Could you check a few things on this model? Use its own coordinates, in mm. A direction names the side the tool comes from. Give positions to 0.01 mm unless a question says otherwise; leave off trailing zeros. Loops run counter-clockwise (first coordinate to the right, second up) from the corner with the lowest first, then second, coordinate; pieces in that order, holes last. Notation, with made-up numbers: M 39,40.5 L 47,40.5 A18 cw 47,75.5 Z; hole C 47,30 d7. An arc over 180 degrees is marked long. Answer in a Markdown table with one row per item. Add a question column.
1. Thinking about a two-plate mould opening in Z: for faces 6 (the flat face through (33, 9, 10)), 7 (the flat face through (3.25, -3.31, 6.04)), 8 (the cylindrical face through (-17.257, -10.412, 5.594)), which applies, released by +Z, released by -Z, zero draft, split by the parting line, or undercut?
2. I'm going to push flat-ended pins straight in: pin 1 Ø3 at (y, z) = (-10, 8) entering from -X; pin 2 Ø5 at (y, z) = (1, 8.5) entering from -X; pin 3 Ø3 at (x, z) = (86, 4.5) entering from +Y. Where does each tip first touch, or does it pass through?
3. Which directions (+Z, -Z, +X, -X, +Y, -Y) give clear straight access to the entire face, cutting with the end or side of a thin tool? Please do faces 1 (the flat face through (-16, -12.947, 5)), 2 (the flat face through (6.1, 10.253, 6.3)), 3 (the flat face through (-19.9, -7.947, 3.8)), 4 (the flat face through (34, 6.053, 5)), 5 (the flat face through (86, -7.947, 3)).
4. If we section it at B-B on x = 17.5: List the corners of the cut face in (y, z) for me, then the cut area to 3 significant figures.
5. If we section it at C-C on y = 8.75: List the corners of the cut face in (x, z) for me, then the cut area to 3 significant figures.
6. I need wall thicknesses on line 1 along X through (y, z) = (-11.1, 5) (3 decimals); line 2 along X through (y, z) = (10.95, 5); line 3 along X through (y, z) = (7.5, 3.75). Which ranges of each line are inside material? Lowest first, please. Write a range as from..to.
7. If we section it at A-A on y = -9.5: List the corners of the cut face in (x, z) for me, then the cut area to 3 significant figures.
8. If we section it at D-D on z = 5: Count the separate pieces of the cut face and the enclosed holes in it, then the cut area to 3 significant figures.
```python
from build123d import *

# Parameters (mm, degrees)
EXTRUDE_1_DEPTH     = 10
SKETCH_2_R          = 1.6
CUT_EXTRUDE_2_DEPTH = 27
SKETCH_3_R          = 3.1
CUT_EXTRUDE_3_DEPTH = 2.8
SKETCH_5_R          = 1.55
CUT_EXTRUDE_4_DEPTH = 6


with BuildPart() as part:
    # 草图1 → 凸台-拉伸1 (new body)
    with BuildSketch(Plane.XY):
        Polygon((-3.188712924, 13.052848472), (33.811287076, 13.052848472), (33.811287076, 6.052848472), (16.311287076, 6.052848472), (-10.188712924, -12.947151528), (-26.188712924, -12.947151528), (-23.688712924, -7.947151528), (-13.688712924, -7.947151528), align=None)
    extrude_1 = extrude(amount=EXTRUDE_1_DEPTH)

    # 镜向1: 凸台-拉伸1 across plane
    add(extrude_1.mirror(Plane(origin=(33.811287076, 13.052848472, 10), x_dir=(0, 0, 1), z_dir=(-1, 0, 0))))

    # 草图2 → 切除-拉伸2 (cut, through all)
    with BuildSketch(Plane(origin=(0, 13.052848472, 0), x_dir=(1, 0, 0), z_dir=(0, 1, 0))):
        with Locations((4.811287076, -5)):
            Circle(SKETCH_2_R)
        with Locations((62.811287076, -5)):
            Circle(SKETCH_2_R)
    extrude(amount=-CUT_EXTRUDE_2_DEPTH, mode=Mode.SUBTRACT)

    # 草图3 → 切除-拉伸3 (cut)
    with BuildSketch(Plane(origin=(0, 13.052848472, 0), x_dir=(1, 0, 0), z_dir=(0, 1, 0))):
        with Locations((4.811287076, -5)):
            Circle(SKETCH_3_R)
        with Locations((62.811287076, -5)):
            Circle(SKETCH_3_R)
    extrude(amount=-CUT_EXTRUDE_3_DEPTH, mode=Mode.SUBTRACT)

    # 草图5 → 切除-拉伸4 (cut, through all)
    with BuildSketch(Plane(origin=(0, -7.947151528, 0), x_dir=(1, 0, 0), z_dir=(0, 1, 0))):
        with Locations((-18.688712924, -5)):
            Circle(SKETCH_5_R)
        with Locations((86.311287076, -5)):
            Circle(SKETCH_5_R)
    extrude(amount=-CUT_EXTRUDE_4_DEPTH, mode=Mode.SUBTRACT)


solid = part.part
```
Results:
| question | item | result |
|---|---|---|
| 1 | face 6 | released by +Z |
| 1 | face 7 | zero draft |
| 1 | face 8 | undercut |
| 2 | pin 1 | x = -25.47 |
| 2 | pin 2 | x = -10.47 |
| 2 | pin 3 | y = -7.95 |
| 3 | face 1 | +Z, -Z, +X, -X, -Y |
| 3 | face 2 | +Y |
| 3 | face 3 | +Z, -Z, -X, +Y |
| 3 | face 4 | +Z, -Z, -Y |
| 3 | face 5 | +Z, -Z, +X, +Y |
| 4 | outline | M 6.05,0 L 13.05,0 L 13.05,10 L 6.05,10 Z |
| 4 | area | 70.0 mm2 |
| 5 | outline | M -5.34,0 L 72.96,0 L 72.96,10 L -5.34,10 Z; hole C 4.81,5 d3.2; hole C 62.81,5 d3.2 |
| 5 | area | 767 mm2 |
| 6 | line 1 | -25.265..-20.239, -17.139..-7.612, 75.235..84.761, 87.861..92.888 |
| 6 | line 2 | -4.24..1.71, 7.91..59.71, 65.91..71.86 |
| 6 | line 3 | -5.97..3.81, 5.81..61.81, 63.81..73.59 |
| 7 | outline | M -24.47,0 L -5.38,0 L -5.38,10 L -24.47,10 Z; M 73,0 L 92.09,0 L 92.09,10 L 73,10 Z; hole C -18.69,5 d3.1; hole C 86.31,5 d3.1 |
| 7 | area | 367 mm2 |
| 8 | separate pieces | 5 |
| 8 | enclosed holes | 0 |
| 8 | area | 1,050 mm2 |
